```python
from build123d import *

# Parameters (mm, degrees)
SKETCH1_W           = 109.1
SKETCH1_H           = 40
BOSS_EXTRUDE1_DEPTH = 8
SKETCH2_W           = 49.3
SKETCH2_H           = 10
BOSS_EXTRUDE2_DEPTH = 8
SKETCH3_W           = 49.3
SKETCH3_H           = 10
BOSS_EXTRUDE3_DEPTH = 8
SKETCH4_R           = 2.75
CUT_EXTRUDE1_DEPTH  = 8
SKETCH5_R           = 5
CUT_EXTRUDE2_DEPTH  = 5.2


with BuildPart() as part:
    # Sketch1 → Boss-Extrude1 (new body)
    with BuildSketch(Plane.XY.offset(238)):
        with Locations((281.75, 300)):
            Rectangle(SKETCH1_W, SKETCH1_H)
        with BuildLine():
            Line((285, 287.25), (291, 287.25))
            ThreePointArc((291, 287.25), (293.75, 290), (291, 292.75))
            Line((291, 292.75), (285, 292.75))
            ThreePointArc((285, 292.75), (282.25, 290), (285, 287.25))
        make_face(mode=Mode.SUBTRACT)
        with BuildLine():
            Line((285, 307.25), (291, 307.25))
            ThreePointArc((291, 307.25), (293.75, 310), (291, 312.75))
            Line((291, 312.75), (285, 312.75))
            ThreePointArc((285, 312.75), (282.25, 310), (285, 307.25))
        make_face(mode=Mode.SUBTRACT)
        with BuildLine():
            Line((305, 287.25), (311, 287.25))
            ThreePointArc((311, 287.25), (313.75, 290), (311, 292.75))
            Line((311, 292.75), (305, 292.75))
            ThreePointArc((305, 292.75), (302.25, 290), (305, 287.25))
        make_face(mode=Mode.SUBTRACT)
        with BuildLine():
            Line((305, 307.25), (311, 307.25))
            ThreePointArc((311, 307.25), (313.75, 310), (311, 312.75))
            Line((311, 312.75), (305, 312.75))
            ThreePointArc((305, 312.75), (302.25, 310), (305, 307.25))
        make_face(mode=Mode.SUBTRACT)
    extrude(amount=BOSS_EXTRUDE1_DEPTH)

    # Sketch2 → Boss-Extrude2 (add)
    with BuildSketch(Plane.XY.offset(238)):
        with Locations((251.85, 275)):
            Rectangle(SKETCH2_W, SKETCH2_H)
    extrude(amount=BOSS_EXTRUDE2_DEPTH)

    # Sketch3 → Boss-Extrude3 (add)
    with BuildSketch(Plane.XY.offset(238)):
        with Locations((251.85, 325)):
            Rectangle(SKETCH3_W, SKETCH3_H)
    extrude(amount=BOSS_EXTRUDE3_DEPTH)

    # Sketch4 → Cut-Extrude1 (cut)
    with BuildSketch(Plane.XY.offset(238)):
        with Locations((252, 281)):
            Circle(SKETCH4_R)
        with Locations((252, 319)):
            Circle(SKETCH4_R)
        with Locations((266, 281)):
            Circle(SKETCH4_R)
        with Locations((266, 319)):
            Circle(SKETCH4_R)
    extrude(amount=CUT_EXTRUDE1_DEPTH, mode=Mode.SUBTRACT)

    # Sketch5 → Cut-Extrude2 (cut)
    with BuildSketch(Plane.XY.offset(238)):
        with Locations((252, 281)):
            Circle(SKETCH5_R)
        with Locations((252, 319)):
            Circle(SKETCH5_R)
        with Locations((266, 281)):
            Circle(SKETCH5_R)
        with Locations((266, 319)):
            Circle(SKETCH5_R)
    extrude(amount=CUT_EXTRUDE2_DEPTH, mode=Mode.SUBTRACT)


solid = part.part
```
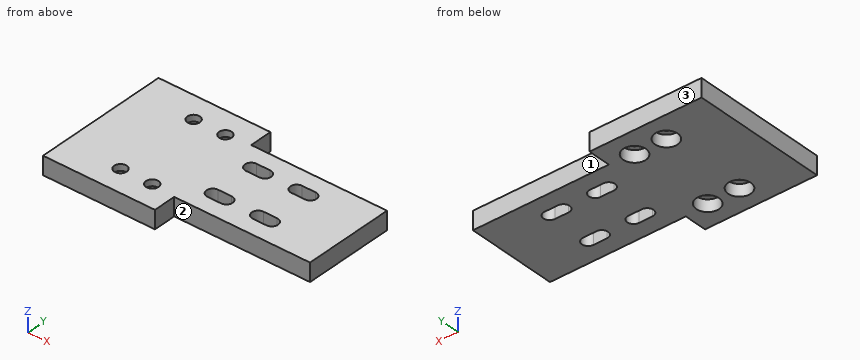
Work out the finished part from the listing and answer in its coordinate system (mm). Face numbers are marked on the shaded views. A direction names the side the tool comes from. Coordinates: 2 decimals unless noted, no trailing zeros. Loops run counter-clockwise (first coordinate to the right, second up) from the corner with the lowest first, then second, coordinate; pieces in that order, holes last. Notation, with made-up numbers: (75.5, 80) -> (97.5, 80) arc R25 ccw to (97.5, 99) -> close; hole circle Ø1 at (-24, 41.5). An arc over 180 degrees is marked (long way). Answer as CSV lines item,"result".
Q1. The part is cut by section C-C on y = 310. Write down the section's boundary in (x, z), and give its area (3 significant figures).
Findings:
outline,"(227.2, 238) -> (282.25, 238) -> (282.25, 246) -> (227.2, 246) -> close; (293.75, 238) -> (302.25, 238) -> (302.25, 246) -> (293.75, 246) -> close; (313.75, 238) -> (336.3, 238) -> (336.3, 246) -> (313.75, 246) -> close"
area,"689 mm²"
Q2. Find the intervals of material crossed by probe 1 along Y at (x, z) = (252, 244.45); probe 2 along Y at (x, z) = (266, 241.1); probe 3 along X at (y, z) = (281, 245.3), in increasing order.
Findings:
probe 1,"y = 270 to 278.25, 283.75 to 316.25, 321.75 to 330"
probe 2,"y = 270 to 276, 286 to 314, 324 to 330"
probe 3,"x = 227.2 to 249.25, 254.75 to 263.25, 268.75 to 336.3"
Q3. The part is cut by section D-D on x = 262. Write down the section's boundary in (y, z).
Findings:
outline,"(270, 238) -> (278, 238) -> (278, 243.2) -> (284, 243.2) -> (284, 238) -> (316, 238) -> (316, 243.2) -> (322, 243.2) -> (322, 238) -> (330, 238) -> (330, 246) -> (270, 246) -> close"
Q4. A tool of negligible diameter and unlimited length cuts with its end or side. For the marked faces 1, 2 and 3, from which of +Z, -Z, +X, -X, +Y, -Y can it reach the whole face along a straight path? Write none if from no direction.
Findings:
face 1,"+Z, -Z, +X, +Y"
face 2,"+Z, -Z, +X, -Y"
face 3,"+Z, -Z, +X, -X, +Y"
Q5. The part is cut by section A-A on z = 239.5. State how many separate pieces and enclosed holes the cut face has, and give its area (3 significant figures).
Findings:
separate pieces,"1"
enclosed holes,"8"
area,"4,810 mm²"
Q6. The part is cut by section B-B on x = 310. Write down the section's boundary in (y, z), and give its area (3 significant figures).
Findings:
outline,"(280, 238) -> (287.25, 238) -> (287.25, 246) -> (280, 246) -> close; (292.75, 238) -> (307.25, 238) -> (307.25, 246) -> (292.75, 246) -> close; (312.75, 238) -> (320, 238) -> (320, 246) -> (312.75, 246) -> close"
area,"232 mm²"
Q7. Each of these flat-tipped pins is pushed along its axis until it touches: pin 1 (5 mm diameter, centred on x = 268, y = 278.5, fed in from -Z); pin 2 (8 mm diameter, centred on x = 266, y = 281, fed in from -Z); pin 3 (4 mm diameter, centred on y = 327, z = 243.5, fed in from +X); pin 4 (3 mm diameter, centred on x = 286.5, z = 242, fed in from -Y). Where does it stop, or does it pass through?
Findings:
pin 1,"stops at z = 238"
pin 2,"stops at z = 243.2"
pin 3,"stops at x = 276.5"
pin 4,"stops at y = 280"
